Part model, mm, in its own coordinate system. Round coordinates to 2 decimals unless told otherwise and drop trailing zeros. Loops run counter-clockwise (first coordinate to the right, second up) from the corner with the lowest first, then second, coordinate; pieces in that order, holes last.
(1) Probe probe 1 along Y at (x, z) = (295, 1.2); probe 2 along Y at (x, z) = (257, 1.2); probe 3 along Y at (x, z) = (319, 1.55). List the from-to ranges inside material, lowest first.
(2) Cut at A-A on x = 290. List the corners of the cut face in (y, z), then the cut area to 3 significant figures.
(3) Mould opens along Y. For faces 1 (the face through (341.56, 54.62, 0.81)), 2 (the face through (253.31, -3.02, 0.79)), 3 (the face through (296, 18, 0)), 4 (the face through (293.202, 25.757, 0.811)) say: +Y half, -Y half, draft (parallel to the pull), parting line (faces both ways), or undercut.
(4) Flat gauge pins, fed straight in: pin 1 (3 mm diameter, centred on x = 342.95, y = -4.32, fed in from +Z); pin 2 (0.5 mm diameter, centred on x = 318, z = 1, fed in from +Y); pin 3 (4.5 mm diameter, centred on x = 294.95, y = 25.68, fed in from -Z); pin 4 (0.8 mm diameter, centred on y = 59, z = 1, fed in from -X). Where does each tip first touch, or does it go through?
(5) Cut at B-B on z = 0.35. Count the separate pieces of the cut face and the enclosed holes in it, then the cut area to 3 significant figures.
(6) Cut at C-C on x = 312.5. List the corners of the cut face in (y, z).
from build123d import *

# Parameters (mm, degrees)
BOSS_EXTRUDE1_DEPTH     = 1.6
SKETCH4_R               = 4
SKETCH4_R_2             = 1.75
CUT_EXTRUDE1_DEPTH      = 1
CUT_EXTRUDE1_DEPTH_BACK = 2.6
SKETCH5_W               = 50
SKETCH5_H               = 120
CUT_EXTRUDE2_DEPTH      = 2.6
SKETCH6_R               = 0.25
CUT_EXTRUDE3_DEPTH      = 2.6


with BuildPart() as part:
    # Sketch3 → Boss-Extrude1 (new body)
    with BuildSketch(Plane.XY):
        with BuildLine():
            Line((254.450402667, 57.180474091), (254.450402667, 62.180474091))
            Line((254.450402667, 62.180474091), (292.450402667, 62.180474091))
            ThreePointArc((292.450402667, 62.180474091), (293.540045449, 62.615149067), (294.031315558, 63.680474091))
            Line((294.031315558, 63.680474091), (307.850402667, 63.680474091))
            Line((307.850402667, 63.680474091), (307.850402667, 58.730474091))
            ThreePointArc((307.850402667, 58.730474091), (308.143295886, 58.02336731), (308.850402667, 57.730474091))
            Line((308.850402667, 57.730474091), (322.050402667, 57.730474091))
            ThreePointArc((322.050402667, 57.730474091), (322.757509449, 58.02336731), (323.050402667, 58.730474091))
            Line((323.050402667, 58.730474091), (323.050402667, 63.680474091))
            Line((323.050402667, 63.680474091), (332.953861053, 63.680474091))
            ThreePointArc((332.953861053, 63.680474091), (333.950402667, 62.76356928), (334.946944282, 63.680474091))
            Line((334.946944282, 63.680474091), (374.453861053, 63.680474091))
            ThreePointArc((374.453861053, 63.680474091), (375.450402667, 62.76356928), (376.446944282, 63.680474091))
            Line((376.446944282, 63.680474091), (390.950402667, 63.680474091))
            ThreePointArc((390.950402667, 63.680474091), (393.071723011, 62.801794434), (393.950402667, 60.680474091))
            Line((393.950402667, 60.680474091), (393.950402667, 58.177015705))
            ThreePointArc((393.950402667, 58.177015705), (393.033497857, 57.180474091), (393.950402667, 56.183932476))
            Line((393.950402667, 56.183932476), (393.950402667, -4.822984295))
            ThreePointArc((393.950402667, -4.822984295), (393.033497857, -5.819525909), (393.950402667, -6.816067524))
            Line((393.950402667, -6.816067524), (393.950402667, -9.319525909))
            ThreePointArc((393.950402667, -9.319525909), (393.071723011, -11.440846253), (390.950402667, -12.319525909))
            Line((390.950402667, -12.319525909), (376.446944282, -12.319525909))
            ThreePointArc((376.446944282, -12.319525909), (375.450402667, -11.402621099), (374.453861053, -12.319525909))
            Line((374.453861053, -12.319525909), (334.946944282, -12.319525909))
            ThreePointArc((334.946944282, -12.319525909), (333.950402667, -11.402621099), (332.953861053, -12.319525909))
            Line((332.953861053, -12.319525909), (293.446944282, -12.319525909))
            ThreePointArc((293.446944282, -12.319525909), (292.450402667, -11.402621099), (291.453861053, -12.319525909))
            Line((291.453861053, -12.319525909), (254.450402667, -12.319525909))
            Line((254.450402667, -12.319525909), (254.450402667, -5.819525909))
            ThreePointArc((254.450402667, -5.819525909), (253.278829792, -2.991098784), (250.450402667, -1.819525909))
            Line((250.450402667, -1.819525909), (245.950402667, -1.819525909))
            Line((245.950402667, -1.819525909), (245.950402667, 53.180474091))
            Line((245.950402667, 53.180474091), (250.450402667, 53.180474091))
            ThreePointArc((250.450402667, 53.180474091), (253.278829792, 54.352046966), (254.450402667, 57.180474091))
        make_face()
    extrude(amount=BOSS_EXTRUDE1_DEPTH)

    # Sketch4 → Cut-Extrude1 (cut, two sides)
    with BuildSketch(Plane.XY.offset(1.6)) as cut_extrude1_sk:
        with Locations((375.450402667, -5.819525909)):
            Circle(SKETCH4_R)
        with Locations((342.950402667, -4.319525909)):
            Circle(SKETCH4_R_2)
        with Locations((294.950402667, 25.680474091)):
            Circle(SKETCH4_R_2)
        with Locations((342.950402667, 55.680474091)):
            Circle(SKETCH4_R_2)
        with Locations((375.450402667, 57.180474091)):
            Circle(SKETCH4_R)
    extrude(amount=CUT_EXTRUDE1_DEPTH, mode=Mode.SUBTRACT)
    extrude(cut_extrude1_sk.sketch, amount=-CUT_EXTRUDE1_DEPTH_BACK, mode=Mode.SUBTRACT)

    # Sketch5 → Cut-Extrude2 (cut, through all)
    with BuildSketch(Plane.XY.offset(1.6)):
        with Locations((370.450402667, 25.680474091)):
            Rectangle(SKETCH5_W, SKETCH5_H)
    extrude(amount=-CUT_EXTRUDE2_DEPTH, mode=Mode.SUBTRACT)

    # Sketch6 → Cut-Extrude3 (cut, through all)
    with BuildSketch(Plane.XY.offset(1.6)):
        with Locations((249.525402667, 49.810474091)):
            Circle(SKETCH6_R)
        with Locations((277.465402667, 49.810474091)):
            Circle(SKETCH6_R)
        with Locations((277.465402667, 47.270474091)):
            Circle(SKETCH6_R)
        with Locations((277.465402667, 4.090474091)):
            Circle(SKETCH6_R)
        with Locations((277.465402667, 1.550474091)):
            Circle(SKETCH6_R)
        with Locations((249.525402667, 1.550474091)):
            Circle(SKETCH6_R)
        with Locations((249.525402667, 4.090474091)):
            Circle(SKETCH6_R)
        with Locations((249.525402667, 6.630474091)):
            Circle(SKETCH6_R)
        with Locations((249.525402667, 9.170474091)):
            Circle(SKETCH6_R)
        with Locations((249.525402667, 11.710474091)):
            Circle(SKETCH6_R)
        with Locations((249.525402667, 14.250474091)):
            Circle(SKETCH6_R)
        with Locations((249.525402667, 16.790474091)):
            Circle(SKETCH6_R)
        with Locations((249.525402667, 19.330474091)):
            Circle(SKETCH6_R)
        with Locations((249.525402667, 21.870474091)):
            Circle(SKETCH6_R)
        with Locations((249.525402667, 24.410474091)):
            Circle(SKETCH6_R)
        with Locations((249.525402667, 26.950474091)):
            Circle(SKETCH6_R)
        with Locations((249.525402667, 29.490474091)):
            Circle(SKETCH6_R)
        with Locations((249.525402667, 32.030474091)):
            Circle(SKETCH6_R)
        with Locations((249.525402667, 34.570474091)):
            Circle(SKETCH6_R)
        with Locations((249.525402667, 37.110474091)):
            Circle(SKETCH6_R)
        with Locations((249.525402667, 39.650474091)):
            Circle(SKETCH6_R)
        with Locations((249.525402667, 42.190474091)):
            Circle(SKETCH6_R)
        with Locations((249.525402667, 44.730474091)):
            Circle(SKETCH6_R)
        with Locations((249.525402667, 47.270474091)):
            Circle(SKETCH6_R)
    extrude(amount=-CUT_EXTRUDE3_DEPTH, mode=Mode.SUBTRACT)


solid = part.part
Final values:
1. probe 1: y = -12.32 to 23.93, 27.43 to 63.68
1. probe 2: y = -12.32 to 62.18
1. probe 3: y = -12.32 to 57.73
2. outline: (-12.32, 0) - (62.18, 0) - (62.18, 1.6) - (-12.32, 1.6) - close
2. area: 119 mm2
3. face 1: undercut
3. face 2: -Y half
3. face 3: draft
3. face 4: undercut
4. pin 1: passes through
4. pin 2: stops at y = 57.73
4. pin 3: stops at z = 0
4. pin 4: stops at x = 254.45
5. separate pieces: 1
5. enclosed holes: 27
5. area: 7,200 mm2
6. outline: (-12.32, 0) - (57.73, 0) - (57.73, 1.6) - (-12.32, 1.6) - close
